Check sheet for the drawn part. Datum: minimum x, y, z corner. Units: mm. Coordinates: 2 decimals unless noted, no trailing zeros. Order: outer loops, then holes, each group sorted by start corner. A loop starts at its lowest first (then second) coordinate and runs counter-clockwise, first axis right, second up.
Q1. Depth check by flat-ended pin: P1, Ø10, axis at x = 115.5, z = 69, coming from the -Y side. Enter the tip coordinate at first touch or a pass-through.
Q2. Cross-section at C-C, the plane y = 2.55. Record the boundary of the cut face in (x, z), and give its area (3 significant figures).
Q3. Cross-section at A-A, the plane x = 60. Record the boundary of the cut face in (y, z), and give its area (3 significant figures).
Q4. Thickness scan on line 1 (X direction, y = 0.85, z = 19); line 2 (Z direction, x = 79, y = 2.7); line 3 (X direction, y = 1.2, z = 4.5) (1 decimal). Record the ranges inside material, lowest first.
Q5. Cross-section at B-B, the plane z = 15. Record the boundary of the cut face in (x, y), and give its area (3 significant figures).
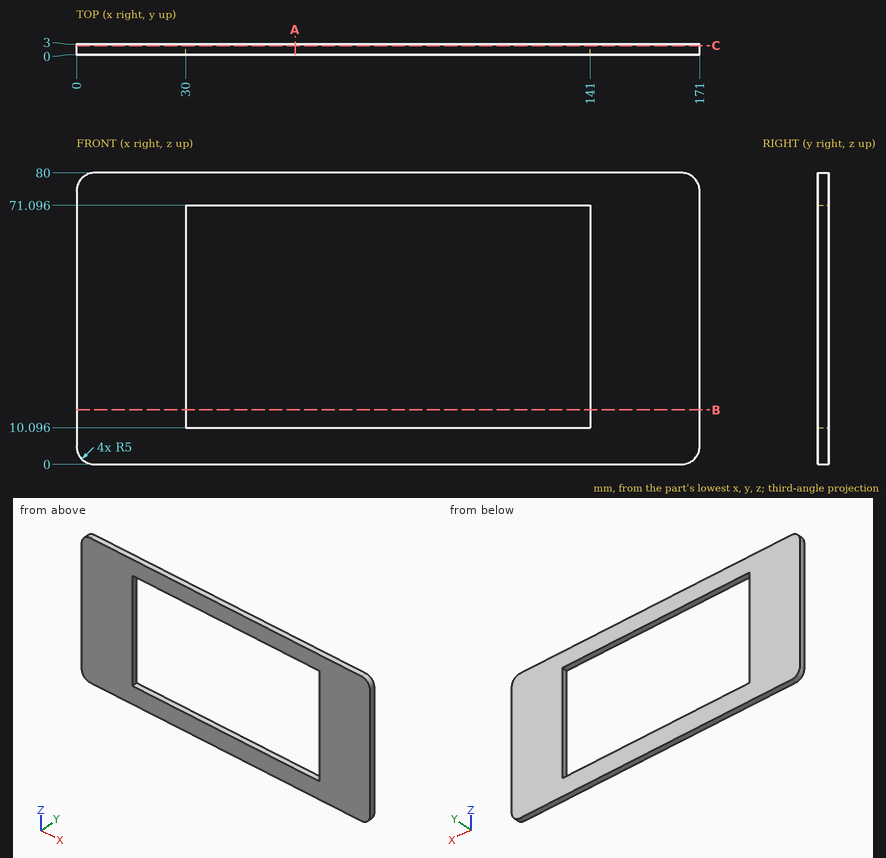
Check values:
1. P1: stops at y = 0
2. outline: (0, 5) arc R5 ccw to (5, 0) - (166, 0) arc R5 ccw to (171, 5) - (171, 75) arc R5 ccw to (166, 80) - (5, 80) arc R5 ccw to (0, 75) - close; hole (30, 10.1) - (141, 10.1) - (141, 71.1) - (30, 71.1) - close
2. area: 6,890 mm2
3. outline: (0, 0) - (3, 0) - (3, 10.1) - (0, 10.1) - close; (0, 71.1) - (3, 71.1) - (3, 80) - (0, 80) - close
3. area: 57.0 mm2
4. line 1: x = 0 to 30, 141 to 171
4. line 2: z = 0 to 10.1, 71.1 to 80
4. line 3: x = 0 to 171
5. outline: (0, 0) - (30, 0) - (30, 3) - (0, 3) - close; (141, 0) - (171, 0) - (171, 3) - (141, 3) - close
5. area: 180 mm2
